```python
from build123d import *

# Parameters (mm, degrees)
EXTRUDE_1_DEPTH     = 20
SKETCH_2_R          = 0.55
CUT_EXTRUDE_1_DEPTH = 29.390183162
SKETCH_3_W          = 16
SKETCH_3_H          = 1.96468827
EXTRUDE_2_DEPTH     = 20
SKETCH_4_W          = 6
SKETCH_4_H          = 20
CUT_EXTRUDE_2_DEPTH = 42.332916665
SKETCH_6_W          = 19.7
SKETCH_6_H          = 1.96468827
EXTRUDE_13_DEPTH    = 17
SKETCH_7_W          = 19.7
SKETCH_7_H          = 1.96468827
EXTRUDE_14_DEPTH    = 17
SKETCH_8_W          = 3
SKETCH_8_H          = 9.85
EXTRUDE_15_DEPTH    = 10
CHAMFER_1_SIZE      = 0.3
SKETCH_10_W         = 3
SKETCH_10_H         = 0.982344135
CUT_EXTRUDE_3_DEPTH = 35.526692573
CHAMFER_3_SIZE      = 0.5
CHAMFER_4_DEPTH     = 20.3
CHAMFER_START       = 20.3
CHAMFER_4_2_DEPTH   = 20.7
CHAMFER_5_SIZE      = 1
CUT_EXTRUDE_4_DEPTH = 49.218253805
CHAMFER_6_SIZE      = 2


with BuildPart() as part:
    # 草图1 → 凸台-拉伸1 (new body)
    with BuildSketch(Plane.XY):
        Polygon((-10, 0.48531173), (-8, 0.48531173), (-8, 2.45), (8, 2.45), (8, 0.48531173), (10, 0.48531173), (10, -2.41468827), (-10, -2.41468827), align=None)
    extrude(amount=EXTRUDE_1_DEPTH)

    # 草图2 → 切除-拉伸1 (cut, through all)
    with BuildSketch(Plane(origin=(10, 0, 0), x_dir=(0, 0, -1), z_dir=(1, 0, 0))):
        with Locations(Location((-2.5, -1.01468827, 0), (0, 0, 90))):
            Circle(SKETCH_2_R)
        with Locations(Location((-18.5, -1.01468827, 0), (0, 0, 90))):
            Circle(SKETCH_2_R)
    extrude(amount=-CUT_EXTRUDE_1_DEPTH, mode=Mode.SUBTRACT)

    # 草图3 → 凸台-拉伸2 (add)
    with BuildSketch(Plane.XY.offset(20)):
        with Locations((0, 1.467655865)):
            Rectangle(SKETCH_3_W, SKETCH_3_H)
    extrude(amount=EXTRUDE_2_DEPTH)

    # 草图4 → 切除-拉伸2 (cut, through all)
    with BuildSketch(Plane.XZ.offset(-0.48531173)):
        with Locations((0, 30)):
            Rectangle(SKETCH_4_W, SKETCH_4_H)
    extrude(amount=-CUT_EXTRUDE_2_DEPTH, mode=Mode.SUBTRACT)

    # 草图6 → 凸台-拉伸13 (add)
    with BuildSketch(Plane.ZY.offset(8)):
        with Locations((30.15, 1.467655865)):
            Rectangle(SKETCH_6_W, SKETCH_6_H)
    extrude(amount=EXTRUDE_13_DEPTH)

    # 草图7 → 凸台-拉伸14 (add)
    with BuildSketch(Plane(origin=(8, 0, 0), x_dir=(0, 0, -1), z_dir=(1, 0, 0))):
        with Locations((-30.15, 1.467655865)):
            Rectangle(SKETCH_7_W, SKETCH_7_H)
    extrude(amount=EXTRUDE_14_DEPTH)

    # 草图8 → 凸台-拉伸15 (add)
    with BuildSketch(Plane(origin=(0, 2.45, 0), x_dir=(1, 0, 0), z_dir=(0, 1, 0))):
        with Locations((-23.5, -25.225)):
            Rectangle(SKETCH_8_W, SKETCH_8_H)
        with Locations((23.5, -25.225)):
            Rectangle(SKETCH_8_W, SKETCH_8_H)
    extrude(amount=EXTRUDE_15_DEPTH)

    # 倒角1
    chamfer_1_edges = [part.edges().sort_by_distance(p)[0] for p in [
        (10, -2.41468827, 10),
        (-10, -2.41468827, 10),
        (-10, 0.48531173, 10),
        (10, 0.48531173, 10),
    ]]
    chamfer(chamfer_1_edges, length=CHAMFER_1_SIZE)

    # 草图10 → 切除-拉伸3 (cut, through all)
    with BuildSketch(Plane(origin=(0, 0, 20.3), x_dir=(-1, 0, 0), z_dir=(0, 0, -1))):
        with Locations((-9.5, 0.976483798)):
            Rectangle(SKETCH_10_W, SKETCH_10_H)
        with Locations((9.5, 0.976483798)):
            Rectangle(SKETCH_10_W, SKETCH_10_H)
    extrude(amount=-CUT_EXTRUDE_3_DEPTH, mode=Mode.SUBTRACT)

    # 倒角3
    chamfer_3_edges = [part.edges().sort_by_distance(p)[0] for p in [
        (3, 2.45, 30),
        (-3, 2.45, 30),
        (-3, 0.48531173, 30),
        (3, 0.48531173, 30),
    ]]
    chamfer(chamfer_3_edges, length=CHAMFER_3_SIZE)

    # 倒角4: read off the stored shape, not the designer's step
    # 倒角4 outline → 倒角4 (cut)
    with BuildSketch(Plane.XY):
        Polygon((-8, 1.45), (-7, 2.45), (-8, 2.45), align=None)
        Polygon((8, 2.45), (7, 2.45), (8, 1.45), align=None)
    extrude(amount=CHAMFER_4_DEPTH, mode=Mode.SUBTRACT)

    # Chamfer 4 2 outline → Chamfer 4 2 (cut)
    with BuildSketch(Plane.XY.offset(CHAMFER_START)):
        Polygon((-8, 1.467655865), (-8, 1.45), (-7.982344135, 1.467655865), align=None)
        Polygon((8, 1.467655865), (7.982344135, 1.467655865), (8, 1.45), align=None)
    extrude(amount=CHAMFER_4_2_DEPTH, mode=Mode.SUBTRACT)

    # 倒角5
    chamfer_5_edges = [part.edges().sort_by_distance(p)[0] for p in [
        (23.5, 12.45, 20.3),
        (22, 12.45, 25.225),
        (23.5, 12.45, 30.15),
        (25, 12.45, 25.225),
        (-23.5, 12.45, 20.3),
        (-25, 12.45, 25.225),
        (-23.5, 12.45, 30.15),
        (-22, 12.45, 25.225),
    ]]
    chamfer(chamfer_5_edges, length=CHAMFER_5_SIZE)

    # 草图11 → 切除-拉伸4 (cut, through all)
    with BuildSketch(Plane(origin=(0, 2.45, 0), x_dir=(1, 0, 0), z_dir=(0, 1, 0))):
        Polygon((-22, -30.15), (-25, -30.15), (-25, -40), (-16, -40), (-16, -30.15), align=None)
        Polygon((16, -30.15), (16, -40), (25, -40), (25, -30.15), (22, -30.15), align=None)
    extrude(amount=-CUT_EXTRUDE_4_DEPTH, mode=Mode.SUBTRACT)

    # 倒角6
    chamfer_6_edges = [part.edges().sort_by_distance(p)[0] for p in [
        (-16, 1.467655865, 40),
        (16, 1.467655865, 40),
    ]]
    chamfer(chamfer_6_edges, length=CHAMFER_6_SIZE)


solid = part.part
```
Geometry check sheet. Reference: the model listing, model coordinates, mm. A direction names the side the tool comes from. Coordinates: 2 decimals unless noted, no trailing zeros. Write each loop counter-clockwise with the first axis right and the second up, starting at its lowest first coordinate (ties: lowest second). Pieces come first, ordered by that corner, then holes. Notation, with made-up numbers: M 61,57.25 L 71,57.25 A24 cw 71,81.25 Z; hole C 23,27 d4. An arc over 180 degrees is marked long. Use one line per item in the form item = value. Start each with the question number.
1) Go/stop test with flat-tipped pins: pin 1 Ø5 at (x, z) = (6, 26.5) entering from -Y; pin 2 Ø5.5 at (x, y) = (-13, 4.5) entering from -Z; pin 3 Ø0.7 at (y, z) = (-0.5, 9) entering from +X. Record where each tip stops, or that it passes through.
2) Set-up check for faces 1 (the flat face through (-22, 7, 25)), 2 (the flat face through (9, 0.485, 10)), 3 (the flat face through (-6, 0.485, 30)): record each of +Z, -Z, +X, -X, +Y, -Y from which the full face is reachable in a straight line by a thin tool's end or side.
3) Section check A-A on y = 4.25. Enter the section's corners in (x, z), and give its area (3 significant figures).
4) Section check D-D on z = 18.5. Enter the section's corners in (x, y).
5) Thickness scan on probe 1 along X at (y, z) = (1, 35.5); probe 2 along X at (y, z) = (6.25, 22); probe 3 along Y at (x, z) = (15, 28.5). Record the ranges inside material, lowest first. Write a range as from..to.
6) Section check C-C on x = -2. Enter the section's corners in (y, z).
Responses:
q1.pin_1 = 0.49
q1.pin_2 = 20.3
q1.pin_3 = 10
q2.face_1 = +Z, -Z, +Y
q2.face_2 = +Z, -Z, +X, +Y
q2.face_3 = +Z, +X, -X, -Y
q3.outline = M -25,20.3 L -22,20.3 L -22,30.15 L -25,30.15 Z; M 22,20.3 L 25,20.3 L 25,30.15 L 22,30.15 Z
q3.area = 59.1 mm2
q4.outline = M -10,-2.11 L -9.7,-2.41 L 9.7,-2.41 L 10,-2.11 L 10,-1.56 L -10,-1.56 Z; M -10,-0.46 L 10,-0.46 L 10,0.19 L 9.7,0.49 L 8,0.49 L 8,1.45 L 7,2.45 L -7,2.45 L -8,1.45 L -8,0.49 L -9.7,0.49 L -10,0.19 Z
q5.probe_1 = -16..-11, -8..-3, 3..8, 11..16
q5.probe_2 = -25..-22, 22..25
q5.probe_3 = 0.49..2.45
q6.outline = M -2.41,0 L 2.45,0 L 2.45,20 L -2.41,20 Z; hole C -1.01,2.5 d1.1; hole C -1.01,18.5 d1.1
